CAD build for the part. Positions are in the model's coordinates, mm. Round coordinates to 2 decimals unless told otherwise and drop trailing zeros. Order: outer loops, then holes, each group sorted by start corner. A loop starts at its lowest first (then second) coordinate and runs counter-clockwise, first axis right, second up. Notation, with made-up numbers: (23.25, 68.25) - (57.25, 68.25) arc R24 cw to (57.25, 99.25) - close; hole circle Ø7 at (-15, 79). An arc over 180 degrees is marked (long way). Use one line per item in the form item = value. Start each with the question number.
from build123d import *

# Parameters (mm, degrees)
SKETCH_2_W          = 620
SKETCH_2_H          = 15
SKETCH_2_R          = 2.6
EXTRUDE_1_DEPTH     = 15
SKETCH_3_W          = 12
SKETCH_3_H          = 12
CUT_EXTRUDE_1_DEPTH = 621.362797079
SKETCH_4_R          = 1.6
CUT_EXTRUDE_2_DEPTH = 621.362797079


with BuildPart() as part:
    # ｽｹｯﾁ2 → ﾎﾞｽ - 押し出し1 (new body)
    with BuildSketch(Plane.XY):
        with Locations((310, 7.5)):
            Rectangle(SKETCH_2_W, SKETCH_2_H)
        with Locations((10, 7.5)):
            Circle(SKETCH_2_R, mode=Mode.SUBTRACT)
        with Locations((610, 7.5)):
            Circle(SKETCH_2_R, mode=Mode.SUBTRACT)
    extrude(amount=EXTRUDE_1_DEPTH)

    # ｽｹｯﾁ3 → ｶｯﾄ - 押し出し1 (cut, through all)
    with BuildSketch(Plane.ZY):
        with Locations((7.5, 7.5)):
            Rectangle(SKETCH_3_W, SKETCH_3_H)
    extrude(amount=-CUT_EXTRUDE_1_DEPTH, mode=Mode.SUBTRACT)

    # ｽｹｯﾁ4 → ｶｯﾄ - 押し出し2 (cut, through all)
    with BuildSketch(Plane(origin=(0, 15, 0), x_dir=(1, 0, 0), z_dir=(0, 1, 0))):
        with Locations(Location((470, -7.5, 0), (0, 0, 270))):
            Circle(SKETCH_4_R)
        with Locations(Location((410, -7.5, 0), (0, 0, 270))):
            Circle(SKETCH_4_R)
        with Locations(Location((150, -7.5, 0), (0, 0, 270))):
            Circle(SKETCH_4_R)
        with Locations(Location((210, -7.5, 0), (0, 0, 270))):
            Circle(SKETCH_4_R)
    extrude(amount=-CUT_EXTRUDE_2_DEPTH, mode=Mode.SUBTRACT)


solid = part.part
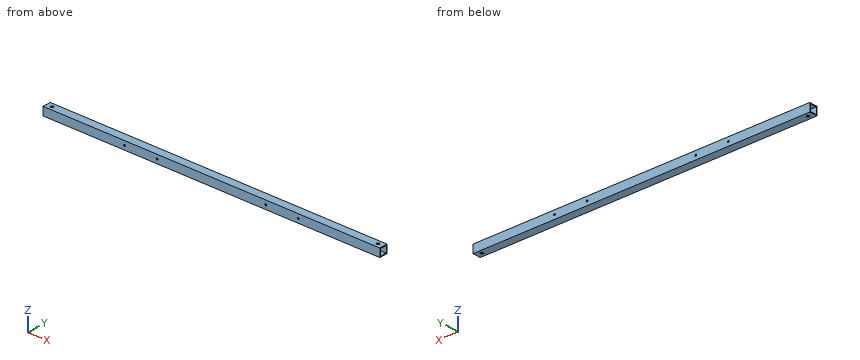
(1) Slice it at B-B (x = 556.5). Give the cut face in (y, z), and give its area (3 significant figures).
(2) Slice it at A-A (y = 7.5). Give the cut face in (x, z).
(3) Wall check: line 1 (X direction, y = 0.6, z = 7.5); line 2 (Z direction, x = 550, y = 11.75). Give the ranges that are in metal, low to high. Write a range as [from, to].
(4) Flat gauge pin, fed straight in: P1, Ø2.5, axis at x = 150, z = 7.5, coming from the +Y side. Where does the tip first touch, or does it go through?
Results list:
q1.outline = (0, 0) - (15, 0) - (15, 15) - (0, 15) - close; hole (1.5, 1.5) - (13.5, 1.5) - (13.5, 13.5) - (1.5, 13.5) - close
q1.area = 81.0 mm²
q2.outline = (0, 0) - (7.4, 0) - (7.4, 1.5) - (0, 1.5) - close; (0, 13.5) - (7.4, 13.5) - (7.4, 15) - (0, 15) - close; (12.6, 0) - (607.4, 0) - (607.4, 1.5) - (12.6, 1.5) - close; (12.6, 13.5) - (607.4, 13.5) - (607.4, 15) - (12.6, 15) - close; (612.6, 0) - (620, 0) - (620, 1.5) - (612.6, 1.5) - close; (612.6, 13.5) - (620, 13.5) - (620, 15) - (612.6, 15) - close
q3.line_1 = [0, 148.4], [151.6, 208.4], [211.6, 408.4], [411.6, 468.4], [471.6, 620]
q3.line_2 = [0, 1.5], [13.5, 15]
q4.P1 = through
